Could you check a few things on this model? Use its own coordinates, in mm. Round coordinates to 2 decimals unless told otherwise and drop trailing zeros. Loops run counter-clockwise (first coordinate to the right, second up) from the corner with the lowest first, then second, coordinate; pieces in that order, holes last.
from build123d import *

# Parameters (mm, degrees)
SKETCH_1_W          = 3
SKETCH_1_H          = 30
EXTRUDE_1_DEPTH     = 76
SKETCH_2_R          = 22.5
EXTRUDE_2_DEPTH     = 3
SKETCH_3_R          = 13
CUT_EXTRUDE_1_DEPTH = 85.801238199
HOLE_WIZARD_M31_D   = 3.4
HOLE_WIZARD_M41_D   = 4.5
FILLET_1_R          = 4
M3X0_51_D           = 2.5


with BuildPart() as part:
    # Эскиз1 → Бобышка-Вытянуть1 (new body)
    with BuildSketch(Plane(origin=(0, 0, 0), x_dir=(1, 0, 0), z_dir=(0, 1, 0))):
        with Locations((1.5, -15)):
            Rectangle(SKETCH_1_W, SKETCH_1_H)
    extrude(amount=EXTRUDE_1_DEPTH)

    # Эскиз2 → Бобышка-Вытянуть2 (add)
    with BuildSketch(Plane.ZY):
        with Locations((15, 46)):
            Circle(SKETCH_2_R)
    extrude(amount=-EXTRUDE_2_DEPTH)

    # Эскиз3 → Вырез-Вытянуть1 (cut, through all)
    with BuildSketch(Plane.ZY):
        with Locations((15, 46)):
            Circle(SKETCH_3_R)
    extrude(amount=-CUT_EXTRUDE_1_DEPTH, mode=Mode.SUBTRACT)

    # Отверстие с зазором M31 (through all)
    with Locations(Plane(origin=(3, -25.024735225, 7.262908886), x_dir=(0, 0, 1), z_dir=(1, 0, 0))):
        with Locations((21.348896652, -84.636540763), (-5.874714424, -84.636540763), (-5.874714424, -57.412929688), (21.348896652, -57.412929688)):
            Hole(HOLE_WIZARD_M31_D / 2)

    # Отверстие с зазором M41 (through all)
    with Locations(Plane(origin=(3, 0, 0), x_dir=(0, 0, -1), z_dir=(1, 0, 0))):
        with Locations((-26, 72), (-4, 72), (-4, 4), (-26, 4)):
            Hole(HOLE_WIZARD_M41_D / 2)

    # Скругление1
    fillet_1_edges = [part.edges().sort_by_distance(p)[0] for p in [
        (1.5, 76, 0),
        (1.5, 0, 0),
        (1.5, 0, 30),
        (1.5, 76, 30),
    ]]
    fillet(fillet_1_edges, radius=FILLET_1_R)

    # Отверстие обработанное метчиком M3x0.51 (through all)
    with Locations(Plane.ZY):
        with Locations((10, 61.12), (20, 61.12), (10, 11.12), (20, 11.12)):
            Hole(M3X0_51_D / 2)


solid = part.part
Item 1: If we section it at B-B, the plane y = 11.12: Please give me the cut outline in (x, z).
Results list:
outline: (0, 0) - (3, 0) - (3, 8.75) - (0, 8.75) - close; (0, 11.25) - (3, 11.25) - (3, 18.75) - (0, 18.75) - close; (0, 21.25) - (3, 21.25) - (3, 30) - (0, 30) - close
Item 2: If we section it at D-D, the plane z = 20: Please give me the cut outline in (x, y), then the cut area to 3 significant figures.
Results list:
outline: (0, 0) - (3, 0) - (3, 9.87) - (0, 9.87) - close; (0, 12.37) - (3, 12.37) - (3, 34) - (0, 34) - close; (0, 58) - (3, 58) - (3, 59.87) - (0, 59.87) - close; (0, 62.37) - (3, 62.37) - (3, 76) - (0, 76) - close
area: 141 mm2
Item 3: If we section it at C-C, the plane y = 51.5: Please give me the cut outline in (x, z).
Results list:
outline: (0, -6.82) - (3, -6.82) - (3, 3.22) - (0, 3.22) - close; (0, 26.78) - (3, 26.78) - (3, 36.82) - (0, 36.82) - close
Item 4: If we section it at A-A, the plane z = 15: Please give me the cut outline in (x, y).
Results list:
outline: (0, 0) - (3, 0) - (3, 33) - (0, 33) - close; (0, 59) - (3, 59) - (3, 76) - (0, 76) - close
Item 5: Will these pins go through, and if not, where does the flat tip stop? pin 1 (4 mm diameter, centred on y = 72, z = 26, fed in from +X) (3 decimals); pin 2 (0.9 mm diameter, centred on x = 1, y = 65.5, fed in from -Z); pin 3 (0.9 mm diameter, centred on x = 1, y = 69, fed in from +Z).
Results list:
pin 1: passes through
pin 2: stops at z = 0
pin 3: stops at z = 30
Item 6: If I drill on line 1 along Y through (x, z) = (0.9, 5.5); line 2 along Y through (x, z) = (2.2, 24); line 3 along Z through (x, y) = (1.3, 5.5), over which ranges is the centre line in solid material (lowest first)?
Results list:
line 1: y = 0 to 2.32, 5.68 to 37.13, 54.87 to 70.32, 73.68 to 76
line 2: y = 0 to 2.97, 5.03 to 36.62, 55.38 to 70.97, 73.03 to 76
line 3: z = 0 to 2.32, 5.68 to 24.32, 27.68 to 30
Item 7: We'd pull the mould along Z, two halves only. Please class faces 1 (the cylindrical face through (1.479, 4.676, 28.146)), 2 (the flat face through (1, 67, 30)), 3 (the flat face through (1, 67, 0)), 4 (the flat face through (1, 76, 15)): released by +Z, released by -Z, zero draft, split by the parting line, or undercut.
Results list:
face 1: undercut
face 2: released by +Z
face 3: released by -Z
face 4: zero draft
